Work out the finished part from the listing and answer in its coordinate system (mm). A direction names the side the tool comes from. Coordinates: 2 decimals unless noted, no trailing zeros. Order: outer loops, then holes, each group sorted by start corner. A loop starts at its lowest first (then second) coordinate and runs counter-clockwise, first axis right, second up. Notation, with made-up numbers: M 54.5,11.5 L 87.5,11.5 A27 cw 87.5,41.5 Z; hole C -11.5,21 d1. An arc over 180 degrees is marked long. Write item = value, one per line. Start each with the question number.
Q1. Find section B-B on z = -2. Give the number of separate pieces and of enclosed holes in the cut face, and give its area (3 significant figures).
Q2. Straight lines are drawn through the part: line 1 along Y through (x, z) = (43, 0); line 2 along X through (y, z) = (-9.5, 23); line 3 along X through (y, z) = (9, 22). For each, find the intervals that lie inside material, in ascending order.
Q3. Determine the mould class of faces 1 (the flat face through (49.284, -15.057, -14.209)), 2 (the conical face through (-4.26, -1.2, -0.27)), 3 (the flat face through (16.51, 10, 21)) for opening direction X: released by +X, released by -X, zero draft, split by the parting line, or undercut.
Q4. Find section A-A on x = 27. Give the vertices of the cut face in (y, z), and give its area (3 significant figures).
Q5. Find section C-C on x = 38. Give the vertices of the cut face in (y, z).
Q6. Each of these flat-tipped pins is pushed along its axis until it touches: P1, Ø5, axis at y = 18, z = 8.5, coming from the -X side; P2, Ø3, axis at x = 26.5, y = 8.5, coming from the -Z side; P3, Ø10, axis at y = -5, z = 0, coming from the -X side. Where does it stop, or does it pass through?
Q7. A tool of negligible diameter and unlimited length cuts with its end or side. For faces 4 (the flat face through (24.13, 10, -21)), 5 (the cylindrical face through (36.435, -6.81, 16.424)), 6 (the flat face through (46.99, -23.1, 0.1)), 7 (the flat face through (49.396, 15.087, 14.401)), from which of +Z, -Z, +X, -X, +Y, -Y can it reach the whole face along a straight path? Write none if from no direction.
Q8. Find section D-D on x = 5.5. Give the vertices of the cut face in (y, z), and give its area (3 significant figures).
```python
from build123d import *

# Parameters (mm, degrees)
F2_R     = 5.08
F3_DEPTH = 63.5
F5_DEPTH = 50


with BuildPart() as f1:
    # F0 (on Front) → F1 (revolve)
    with BuildSketch(Plane.XZ):
        Polygon((0, 25.3715255082), (0, 0), (19.05, 0), (19.05, 17.78), (53.34, 17.78), (53.34, 25.3715255082), (49.53, 25.3715255082), (49.53, 22.86), (46.99, 22.86), (46.99, 25.3715255082), (44.45, 25.3715255082), (44.45, 22.86), (41.91, 22.86), (41.91, 25.3715255082), (24.13, 25.3715255082), (24.13, 22.86), (21.59, 22.86), (21.59, 25.3715255082), (19.05, 25.3715255082), (19.05, 22.86), (16.51, 22.86), (16.51, 25.3715255082), (13.97, 25.3715255082), (13.97, 22.86), (11.43, 22.86), (11.43, 25.3715255082), (8.89, 25.3715255082), (8.89, 22.86), (6.35, 22.86), (6.35, 25.3715255082), align=None)
        Polygon((-4.47870531, 0), (0, 0), (0, 25.3715255082), (0, 25.4), align=None)
    revolve(axis=Axis((9.525, 0, 0), (-1, 0, 0)))

    # F2 (on Front) → F3 (cut, symmetric)
    with BuildSketch(Plane.XZ):
        with Locations((31.115, 0)):
            Circle(F2_R)
    extrude(amount=F3_DEPTH, both=True, mode=Mode.SUBTRACT)

    # F4 (on Top) → F5 (cut, symmetric)
    with BuildSketch(Plane.XY):
        Polygon((53.34, -16.1435935394), (53.34, 16.1435935394), (45.34, 14), (45.34, -14), align=None)
    extrude(amount=F5_DEPTH, both=True, mode=Mode.SUBTRACT)


solid = f1.part
```
Findings below:
q1.separate_pieces = 3
q1.enclosed_holes = 0
q1.area = 1,380 mm^2
q2.line_1 = -22.86 to -17.78, 17.78 to 22.86
q2.line_2 = -0.09 to 6.35, 8.89 to 11.43, 13.97 to 16.51, 19.05 to 21.59, 24.13 to 41.91, 44.45 to 45.34
q2.line_3 = -0.29 to 6.35, 8.89 to 11.43, 13.97 to 16.51, 19.05 to 21.59, 24.13 to 41.91, 44.45 to 45.34
q3.face_1 = released by +X
q3.face_2 = released by -X
q3.face_3 = undercut
q4.outline = M -25.2,-2.98 A25.37 ccw 25.2,-2.98 L 17.53,-2.98 A17.78 cw -17.53,-2.98 Z; M -25.2,2.98 L -17.53,2.98 A17.78 cw 17.53,2.98 L 25.2,2.98 A25.37 ccw Z
q4.area = 938 mm^2
q5.outline = C 0,0 d50.74; hole C 0,0 d35.56
q6.P1 = -1.41
q6.P2 = -24.39
q6.P3 = -4.48
q7.face_4 = none
q7.face_5 = +X
q7.face_6 = -Y
q7.face_7 = +Z, -Z, +X
q8.outline = C 0,0 d50.74
q8.area = 2,020 mm^2
